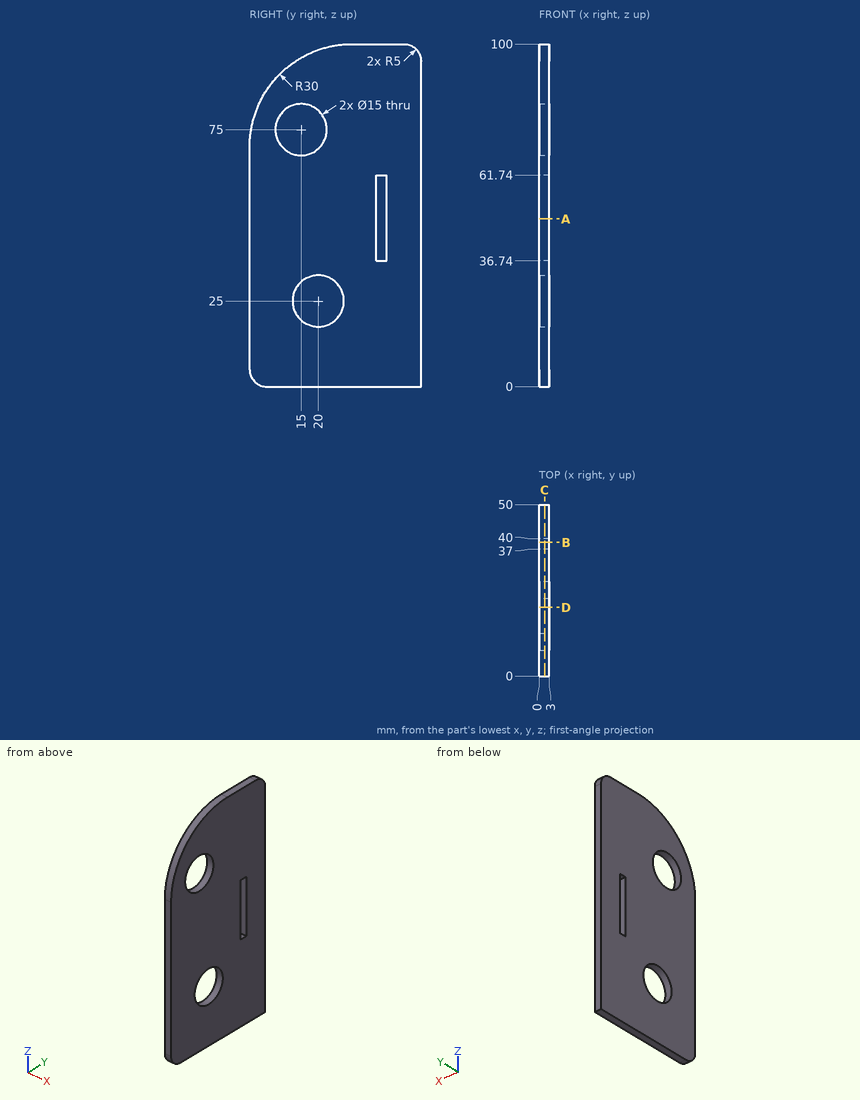
Study the drawing (mm; zero at the part's minimum x, y, z) and answer. Coordinates: 2 decimals unless noted, no trailing zeros. Write each loop counter-clockwise with the first axis right and the second up, starting at its lowest first coordinate (ties: lowest second). Pieces come first, ordered by that corner, then holes.
Q1. Section D-D, the plane y = 20 is taken. Write down the section's boundary in (x, z) (1 decimal).
Returned:
outline: (0, 0) - (3, 0) - (3, 17.5) - (0, 17.5) - close; (0, 32.5) - (3, 32.5) - (3, 69.4) - (0, 69.4) - close; (0, 80.6) - (3, 80.6) - (3, 98.3) - (0, 98.3) - close
Q2. Section C-C, the plane x = 1.6 is taken. Write down the section's boundary in (y, z), then the cut area to 3 significant figures.
Returned:
outline: (0, 5) arc R5 ccw to (5, 0) - (50, 0) - (50, 95) arc R5 ccw to (45, 100) - (30, 100) arc R30 ccw to (0, 70) - close; hole circle Ø15 at (15, 75); hole circle Ø15 at (20, 25); hole (37, 36.74) - (40, 36.74) - (40, 61.74) - (37, 61.74) - close
area: 4,370 mm2
Q3. Section B-B, the plane y = 39 is taken. Write down the section's boundary in (x, z), then the cut area to 3 significant figures.
Returned:
outline: (0, 0) - (3, 0) - (3, 36.74) - (0, 36.74) - close; (0, 61.74) - (3, 61.74) - (3, 100) - (0, 100) - close
area: 225 mm2
Q4. Find the intervals of material crossed by line 1 along Z through (x, y) = (2.6, 17.5); line 2 along Z through (x, y) = (2.45, 15); line 3 along Y through (x, z) = (1, 61), in increasing order.
Returned:
line 1: z = 0 to 17.93, 32.07 to 67.93, 82.07 to 97.27
line 2: z = 0 to 19.41, 30.59 to 67.5, 82.5 to 95.98
line 3: y = 0 to 37, 40 to 50
Q5. Section A-A, the plane z = 49 is taken. Write down the section's boundary in (x, y).
Returned:
outline: (0, 0) - (3, 0) - (3, 37) - (0, 37) - close; (0, 40) - (3, 40) - (3, 50) - (0, 50) - close
Q6. Given P1, Ø12, axis at y = 20, z = 25, coming from the +X side; P2, Ø1.5, axis at x = 0.5, z = 77.5, coming from the -Y side, each flat-ended and moving along its own axis, determine where each tip first touches the part or whether it passes through.
Returned:
P1: passes through
P2: stops at y = 0.77
